The listing builds one solid part. Answer for the finished solid, in the listing's coordinates (mm). Coordinates: 2 decimals unless noted, no trailing zeros. Order: outer loops, then holes, each group sorted by start corner. A loop starts at its lowest first (then second) coordinate and runs counter-clockwise, first axis right, second up. Notation, with made-up numbers: (75.25, 42.25) -> (125.25, 42.25) arc R22 ccw to (125.25, 49.25) -> close; hole circle Ø1 at (88.25, -18). An arc over 180 degrees is marked (long way). Return JSON: item names as keys, results as strings.
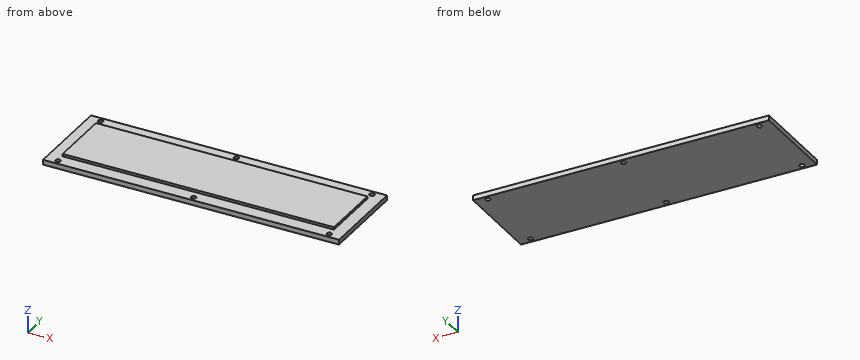
```python
from build123d import *

# Parameters (mm, degrees)
SKETCH1_W           = 120
SKETCH1_H           = 36
BOSS_EXTRUDE1_DEPTH = 2
SKETCH2_W           = 110
SKETCH2_H           = 25
BOSS_EXTRUDE2_DEPTH = 1
SKETCH3_R           = 1
CUT_EXTRUDE1_DEPTH  = 63.673758464
SKETCH4_R           = 1
CUT_EXTRUDE2_DEPTH  = 10


with BuildPart() as part:
    # Sketch1 → Boss-Extrude1 (new body)
    with BuildSketch(Plane.XY):
        Rectangle(SKETCH1_W, SKETCH1_H)
    extrude(amount=BOSS_EXTRUDE1_DEPTH)

    # Sketch2 → Boss-Extrude2 (add)
    with BuildSketch(Plane.XY.offset(2)):
        Rectangle(SKETCH2_W, SKETCH2_H)
    extrude(amount=BOSS_EXTRUDE2_DEPTH)

    # Sketch3 → Cut-Extrude1 (cut, through all)
    with BuildSketch(Plane.XY.offset(2)):
        with Locations((-55, 16)):
            Circle(SKETCH3_R)
        with Locations((-55, -16)):
            Circle(SKETCH3_R)
        with Locations((55, 16)):
            Circle(SKETCH3_R)
        with Locations((55, -16)):
            Circle(SKETCH3_R)
    extrude(amount=-CUT_EXTRUDE1_DEPTH, mode=Mode.SUBTRACT)

    # Sketch4 → Cut-Extrude2 (cut)
    with BuildSketch(Plane(origin=(0, 0, 0), x_dir=(-1, 0, 0), z_dir=(0, 0, -1))):
        with Locations((0, 16)):
            Circle(SKETCH4_R)
        with Locations((0, -16)):
            Circle(SKETCH4_R)
    extrude(amount=-CUT_EXTRUDE2_DEPTH, mode=Mode.SUBTRACT)


solid = part.part
```
Item 1: Flat-ended cylindrical pins translate along their axes: pin 1 (0.5 mm diameter, centred on y = 0, z = 2.5, fed in from +X); pin 2 (0.5 mm diameter, centred on x = 18.5, z = 2.5, fed in from -Y); pin 3 (0.8 mm diameter, centred on y = -2, z = 2.5, fed in from -X). Find the tip coordinate at first contact, or state that the pin passes through.
Answer list:
{"pin 1": "x = 55", "pin 2": "y = -12.5", "pin 3": "x = -55"}
Item 2: The part is cut by section A-A on x = 37.5. Determine the outline of the cut face in (y, z).
Answer list:
{"outline": "(-18, 0) -> (18, 0) -> (18, 2) -> (12.5, 2) -> (12.5, 3) -> (-12.5, 3) -> (-12.5, 2) -> (-18, 2) -> close"}
Item 3: Find the intervals of material crossed by probe 1 along Y at (x, z) = (-55, 0.9); probe 2 along Z at (x, y) = (23, -15); probe 3 along Y at (x, z) = (-17.5, 2.95), in increasing order.
Answer list:
{"probe 1": "-18 to -17, -15 to 15, 17 to 18", "probe 2": "0 to 2", "probe 3": "-12.5 to 12.5"}
